from build123d import *

# Parameters (mm, degrees)
F1_DEPTH = 20


with BuildPart() as f1:
    # F0 (on Top) → F1 (new body)
    with BuildSketch(Plane.XY):
        with BuildLine():
            ThreePointArc((6.614378, -7.5), (9.114378, -4.114378), (10, 0))
            ThreePointArc((10, 0), (9.114378, 4.114378), (6.614378, 7.5))
            Line((6.614378, 7.5), (-6.614378, 7.5))
            ThreePointArc((-6.614378, 7.5), (-10, 0), (-6.614378, -7.5))
            Line((-6.614378, -7.5), (6.614378, -7.5))
        make_face()
    extrude(amount=F1_DEPTH)


solid = f1.part
Model file for the job. Use its own axes, mm. Give positions to 0.01 mm unless a question says otherwise; leave off trailing zeros. Loops run counter-clockwise (first coordinate to the right, second up) from the corner with the lowest first, then second, coordinate; pieces in that order, holes last.
1) Saw through at B-B (y = -6). Write the cut outline in (x, z), plus the area to 3 significant figures.
2) Wall check: line 1 (X direction, y = -6.5, z = 17.75); line 2 (Y direction, x = 8.25, z = 1.75); line 3 (X direction, y = -6, z = 14.75). Give the ranges that are in metal, low to high.
3) Saw through at A-A (z = 11). Write the cut outline in (x, y), plus the area to 3 significant figures.
4) Saw through at C-C (y = -3.75). Write the cut outline in (x, z), plus the area to 3 significant figures.
Answer block:
1. outline: (-8, 0) - (8, 0) - (8, 20) - (-8, 20) - close
1. area: 320 mm2
2. line 1: x = -7.6 to 7.6
2. line 2: y = -5.65 to 5.65
2. line 3: x = -8 to 8
3. outline: (-6.61, -7.5) - (6.61, -7.5) arc R10 ccw to (10, 0) arc R10 ccw to (6.61, 7.5) - (-6.61, 7.5) arc R10 ccw to start
3. area: 269 mm2
4. outline: (-9.27, 0) - (9.27, 0) - (9.27, 20) - (-9.27, 20) - close
4. area: 371 mm2
